Here's how the part is built. I have some questions about the finished solid (model axes, mm). A direction names the side the tool comes from. Coordinates: 2 decimals unless noted, no trailing zeros. Loops run counter-clockwise (first coordinate to the right, second up) from the corner with the lowest first, then second, coordinate; pieces in that order, holes last. Notation, with made-up numbers: M 71,-35.75 L 107,-35.75 A22 ccw 107,0.25 Z; hole C -33,56.25 d8. An arc over 180 degrees is marked long. Use CSV: the item, a comma, the result in double quotes. Start each with the question number.
Q1. If we section it at B-B (z = 10.25): Please give me the cut outline in (x, y) (3 decimals).
Q2. Please list where these lines run through material, in increasing order: probe 1 along X at (y, z) = (21, 10.5); probe 2 along X at (y, z) = (-22, 9.25); probe 3 along X at (y, z) = (-32, 22). Write a range as [from, to].
Q3. For pin 1 Ø6 at (x, y) = (-1, -46.5) entering from +Z; pin 2 Ø5 at (x, y) = (38.97, -22.5) entering from +Z; pin 3 Ø1 at (x, z) = (13.5, 15.5) entering from +Y; pin 4 Ø2 at (x, z) = (-30.5, 20) entering from +Y, each with a flat end and sliding along its axis, tell me the tip position at first contact or that it passes through.
Q4. If we section it at A-A (y = 0): Please give me the cut outline in (x, z), and give its area (3 significant figures).
Q5. If we mould it in two halves opening along X, with no side actions, what happens to faces 1 (the cylindrical face through (28, 45, 16)), 2 (the flat face through (-35, 16, 24)), 3 (the flat face through (-40, -20, 20)), 4 (the flat face through (-40, 25, 20))? For each: +X half, -X half, draft (parallel to the pull), parting line (faces both ways), or undercut.
Q6. If we section it at D-D (z = 22): Please give me the cut outline in (x, y) (3 decimals).
Q7. Which directions (+Z, -Z, +X, -X, +Y, -Y) give clear straight access to the entire face, cutting with the end or side of a thin tool? Please do faces 5 (the cylindrical face through (-4.686, 35.694, 19.447)), 6 (the cylindrical face through (-41.19, 25.4, 21.97)), 7 (the flat face through (-33, 15, 15.75)).
Q8. If we section it at C-C (x = 0): State how many separate pieces and enclosed holes the cut face has, and give its area (3 significant figures).
from build123d import *

# Parameters (mm, degrees)
CYLINDER014005880_R                            = 40.05
CYLINDER014005880_DEPTH                        = 16
CYLINDER014005882_R                            = 3.65
CYLINDER014005882_DEPTH                        = 4
CYLINDER014005881_R                            = 2.15
CYLINDER014005881_DEPTH                        = 24
FUSION001089102007007003008015_PLACEMENT_ANGLE = 60
FUSION001089102007007003008011_PLACEMENT_ANGLE = 120
FUSION001089102007007003008009_PLACEMENT_ANGLE = 180
FUSION001089102007007003008012_PLACEMENT_ANGLE = 240
FUSION001089102007007003008014_PLACEMENT_ANGLE = 60
FUSION001089102007007003008010_PLACEMENT_ANGLE = 30
CYLINDER014005879_R                            = 36
CYLINDER014005879_DEPTH                        = 16
CYLINDER014005878_R                            = 53
CYLINDER014005878_DEPTH                        = 16
CHAMFER013_SIZE                                = 0.75


with BuildPart() as obj1:
    # Cylinder014005880 → Cylinder014005880 (new body)
    with BuildSketch(Plane.XY.offset(-0.25)):
        Circle(CYLINDER014005880_R)
    extrude(amount=CYLINDER014005880_DEPTH)


with BuildPart() as obj2:
    # Cylinder014005882 → Cylinder014005882 (new body)
    with BuildSketch(Plane(origin=(45, 0, 4), x_dir=(1, 0, 0), z_dir=(0, 0, 1))):
        Circle(CYLINDER014005882_R)
    extrude(amount=CYLINDER014005882_DEPTH)


with BuildPart() as obj3:
    # Cylinder014005881 → Cylinder014005881 (new body)
    with BuildSketch(Plane(origin=(45, 0, -16), x_dir=(1, 0, 0), z_dir=(0, 0, 1))):
        Circle(CYLINDER014005881_R)
    extrude(amount=CYLINDER014005881_DEPTH)

    # Fusion001089102007007003008013: union obj2
    add(obj2.part)


with BuildPart() as obj4:
    # Fusion001089102007007003008015 base: copy of obj3
    add(obj3.part)


with BuildPart() as obj4_1:
    # Fusion001089102007007003008015 placement: moved
    add(obj4.part.rotate(Axis((0, 0, 0), (0, 0, 1)), FUSION001089102007007003008015_PLACEMENT_ANGLE))


with BuildPart() as obj5:
    # Fusion001089102007007003008011 base: copy of obj3
    add(obj3.part)


with BuildPart() as obj5_1:
    # Fusion001089102007007003008011 placement: moved
    add(obj5.part.rotate(Axis((0, 0, 0), (0, 0, 1)), FUSION001089102007007003008011_PLACEMENT_ANGLE))


with BuildPart() as obj6:
    # Fusion001089102007007003008009 base: copy of obj3
    add(obj3.part)


with BuildPart() as obj6_1:
    # Fusion001089102007007003008009 placement: moved
    add(obj6.part.rotate(Axis((0, 0, 0), (0, 0, 1)), FUSION001089102007007003008009_PLACEMENT_ANGLE))


with BuildPart() as obj7:
    # Fusion001089102007007003008012 base: copy of obj3
    add(obj3.part)


with BuildPart() as obj7_1:
    # Fusion001089102007007003008012 placement: moved
    add(obj7.part.rotate(Axis((0, 0, 0), (0, 0, 1)), FUSION001089102007007003008012_PLACEMENT_ANGLE))


with BuildPart() as obj8:
    # Fusion001089102007007003008014 base: copy of obj3
    add(obj3.part)


with BuildPart() as obj8_1:
    # Fusion001089102007007003008014 placement: moved
    add(obj8.part.rotate(Axis((0, 0, 0), (0, 0, -1)), FUSION001089102007007003008014_PLACEMENT_ANGLE))


with BuildPart() as fusion001089102007007003008010:
    # Fusion001089102007007003008010 base: copy of obj3
    add(obj3.part)

    # Fusion001089102007007003008010: union obj4, obj5, obj6, obj7, obj8
    add(obj4_1.part)
    add(obj5_1.part)
    add(obj6_1.part)
    add(obj7_1.part)
    add(obj8_1.part)


with BuildPart() as fusion001089102007007003008010_1:
    # Fusion001089102007007003008010 placement: moved
    add(fusion001089102007007003008010.part.moved(Location((0, 0, 16))).rotate(Axis((0, 0, 16), (0, 0, 1)), FUSION001089102007007003008010_PLACEMENT_ANGLE))


with BuildPart() as fusion001089102007007003008016:
    # Cylinder014005879 → Cylinder014005879 (new body)
    with BuildSketch(Plane.XY.offset(8)):
        Circle(CYLINDER014005879_R)
    extrude(amount=CYLINDER014005879_DEPTH)

    # Fusion001089102007007003008016: union obj1, Fusion001089102007007003008010
    add(obj1.part)
    add(fusion001089102007007003008010_1.part)


with BuildPart() as obj9:
    # Cylinder014005878 → Cylinder014005878 (new body)
    with BuildSketch(Plane.XY.offset(8)):
        Circle(CYLINDER014005878_R)
    extrude(amount=CYLINDER014005878_DEPTH)

    # Cut009003003009003002: cut Fusion001089102007007003008016
    add(fusion001089102007007003008016.part, mode=Mode.SUBTRACT)

    # Chamfer013
    chamfer013_edges = [obj9.edges().sort_by_distance(p)[0] for p in [
        (-53, 0, 24),
        (-53, 0, 8),
        (-36, 0, 24),
        (-40.05, 0, 8),
    ]]
    chamfer(chamfer013_edges, length=CHAMFER013_SIZE)


solid = obj9.part
Results below:
1,outline,"C 0,0 d106; hole C -38.971,-22.5 d4.3; hole C -38.971,22.5 d4.3; hole C 0,0 d80.1; hole C 0,-45 d4.3; hole C 0,45 d4.3; hole C 38.971,-22.5 d4.3; hole C 38.971,22.5 d4.3"
2,probe 1,"[-48.66, -40.51], [-37.43, -34.1], [34.1, 37.43], [40.51, 48.66]"
2,probe 2,"[-48.22, -41.06], [-36.88, -33.47], [33.47, 36.88], [41.06, 48.22]"
2,probe 3,"[-42.25, -16.49], [16.49, 42.25]"
3,pin 1,"z = 24"
3,pin 2,"z = 20"
3,pin 3,"y = 51.38"
3,pin 4,"y = 44.03"
4,outline,"M -53,8.75 L -52.25,8 L -40.8,8 L -40.05,8.75 L -40.05,15.75 L -36,15.75 L -36,23.25 L -36.75,24 L -52.25,24 L -53,23.25 Z; M 36,15.75 L 40.05,15.75 L 40.05,8.75 L 40.8,8 L 52.25,8 L 53,8.75 L 53,23.25 L 52.25,24 L 36.75,24 L 36,23.25 Z"
4,area,"479 mm^2"
5,face 1,"parting line"
5,face 2,"draft"
5,face 3,"undercut"
5,face 4,"undercut"
6,outline,"C 0,0 d106; hole C -38.971,-22.5 d7.3; hole C -38.971,22.5 d7.3; hole C 0,0 d72; hole C 0,-45 d7.3; hole C 0,45 d7.3; hole C 38.971,-22.5 d7.3; hole C 38.971,22.5 d7.3"
7,face 5,"+Z, -Z"
7,face 6,"+Z"
7,face 7,"-Z"
8,separate pieces,"4"
8,enclosed holes,"0"
8,area,"317 mm^2"
